Input: part model. Units: mm. Frame: model coordinates. A direction names the side the tool comes from. Give positions to 0.01 mm unless a question says otherwise; leave off trailing zeros. Order: outer loops, then holes, each group sorted by start corner. A loop starts at its lowest first (then second) coordinate and runs counter-clockwise, first axis right, second up. Notation, with made-up numbers: (61.25, -20.5) - (73.25, -20.5) arc R18 cw to (73.25, -8.5) - close; hole circle Ø11 at (-26, 77.5). An arc over 180 degrees is marked (long way). Answer in a Markdown table with one row per item. Add a question column.
1. Section query C-C on z = 23.5. Return loops of the section in (x, y).
2. Section query D-D on y = -37.5. Return loops of the section in (x, z), and give its area (3 significant figures).
3. Ray query, line 1 (Y direction, x = 65, z = 1.95); line 2 (Z direction, x = -8, y = 39.5); line 3 (X direction, y = -38.5, z = 9). Return the intervals inside material, ascending. Write a range as [from, to].
4. Mould query, pull axis X, two halves, no side actions, for faces 1 (the face through (85, 6, 2)), 2 (the face through (-7, -85, 2)), 3 (the face through (59.5, 70.1, 3)). Classes: released by +X, released by -X, zero draft, split by the parting line, or undercut.
5. Section query A-A on y = 65. Return loops of the section in (x, z).
6. Access query for faces 4 (the face through (-45, -60, 26)), 5 (the face through (60, 42, 26)), 6 (the face through (60, 45, 26)). Directions: +Z, -Z, +X, -X, +Y, -Y. A direction counts if a zero-diameter tool reaches every point of the face in a straight line with its end or side. Return the directions, or none.
7. Contact query for flat-ended pins moving along their axis: pin 1 (6 mm diameter, centred on y = 15.5, z = 11.5, fed in from -X); pin 2 (1.5 mm diameter, centred on x = -44, z = 33.5, fed in from +Y); pin 3 (3 mm diameter, centred on x = -26.5, y = -16, fed in from +Z); pin 4 (5 mm diameter, centred on x = 60.5, y = -46.5, fed in from -Z). Output: stop coordinate, or through.
```python
from build123d import *

# Parameters (mm, degrees)
F0_W     = 170
F0_H     = 170
F0_R     = 7.5
F1_DEPTH = 6
F2_W     = 3
F2_H     = 50
F2_W_2   = 50
F2_H_2   = 3
F3_DEPTH = 40


with BuildPart() as f1:
    # F0 (on Top) → F1 (new body)
    with BuildSketch(Plane.XY):
        Rectangle(F0_W, F0_H)
        with Locations((-65, -65)):
            Circle(F0_R, mode=Mode.SUBTRACT)
        with Locations((65, -65)):
            Circle(F0_R, mode=Mode.SUBTRACT)
        with Locations((-65, 65)):
            Circle(F0_R, mode=Mode.SUBTRACT)
        with Locations((65, 65)):
            Circle(F0_R, mode=Mode.SUBTRACT)
    extrude(amount=F1_DEPTH)

    # F2 (on face) → F3 (join)
    with BuildSketch(Plane.XY.offset(6)):
        with Locations((-43.5, -60)):
            Rectangle(F2_W, F2_H)
        with Locations((60, 43.5)):
            Rectangle(F2_W_2, F2_H_2)
    extrude(amount=F3_DEPTH)


solid = f1.part
```
Answer:
| question | item | result |
|---|---|---|
| 1 | outline | (-45, -85) - (-42, -85) - (-42, -35) - (-45, -35) - close; (35, 42) - (85, 42) - (85, 45) - (35, 45) - close |
| 2 | outline | (-85, 0) - (85, 0) - (85, 6) - (-42, 6) - (-42, 46) - (-45, 46) - (-45, 6) - (-85, 6) - close |
| 2 | area | 1,140 mm² |
| 3 | line 1 | y = [-85, -72.5], [-57.5, 57.5], [72.5, 85] |
| 3 | line 2 | z = [0, 6] |
| 3 | line 3 | x = [-45, -42] |
| 4 | face 1 | released by +X |
| 4 | face 2 | zero draft |
| 4 | face 3 | undercut |
| 5 | outline | (-85, 0) - (-72.5, 0) - (-72.5, 6) - (-85, 6) - close; (-57.5, 0) - (57.5, 0) - (57.5, 6) - (-57.5, 6) - close; (72.5, 0) - (85, 0) - (85, 6) - (72.5, 6) - close |
| 6 | face 4 | +Z, -X, +Y, -Y |
| 6 | face 5 | +Z, +X, -X, -Y |
| 6 | face 6 | +Z, +X, -X, +Y |
| 7 | pin 1 | passes through |
| 7 | pin 2 | stops at y = -35 |
| 7 | pin 3 | stops at z = 6 |
| 7 | pin 4 | stops at z = 0 |
